Answer from the drawing. Dimensions are ordinates in mm from the lowest x, y and z of the part. A direction names the side the tool comes from. Give positions to 0.01 mm unless a question says otherwise; leave off trailing zeros. Order: outer loops, then holes, each group sorted by start corner. A loop starts at its lowest first (then second) coordinate and runs counter-clockwise, first axis right, second up.
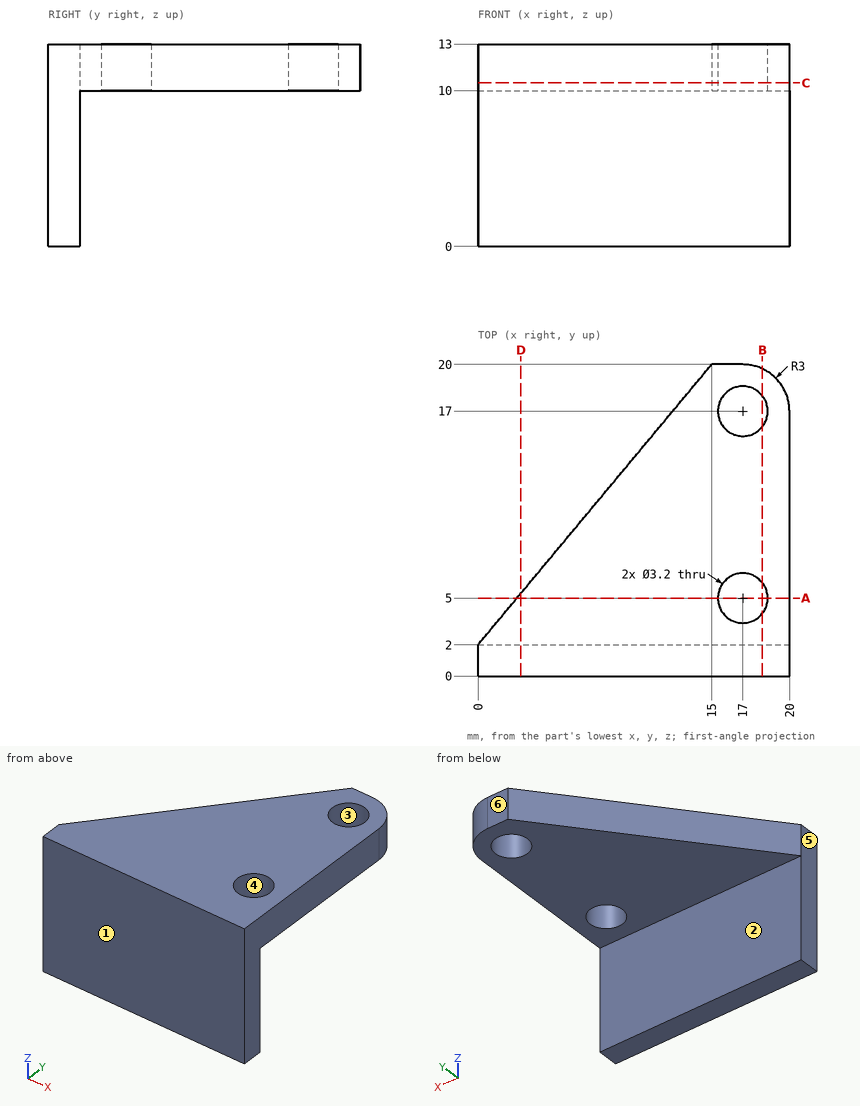
1) Consider L1, parallel to Y at x = 17, z = 12.2; L2, parallel to Y at x = 5.5, z = 4; L3, parallel to Z at x = 13, y = 11.5. Determine where each line is inside the solid, lowest interval first.
Final values:
L1: y = 0 to 3.4, 6.6 to 15.4, 18.6 to 20
L2: y = 0 to 2
L3: z = 10 to 13
2) The part is cut by section A-A on y = 5. Determine the outline of the cut face in (x, z), and give its area (3 significant figures).
Final values:
outline: (2.5, 10) - (15.4, 10) - (15.4, 13) - (2.5, 13) - close; (18.6, 10) - (20, 10) - (20, 13) - (18.6, 13) - close
area: 42.9 mm2
3) A tool of negligible diameter and unlimited length cuts with its end or side. For the marked faces 1 and 2, from which of +Z, -Z, +X, -X, +Y, -Y can it reach the whole face along a straight path? Write none if from no direction.
Final values:
face 1: +Z, -Z, +X, -X, -Y
face 2: -Z, +X, -X, +Y
4) The part is cut by section B-B on x = 18.25. Determine the outline of the cut face in (y, z).
Final values:
outline: (0, 0) - (2, 0) - (2, 10) - (4, 10) - (4, 13) - (0, 13) - close; (6, 10) - (16, 10) - (16, 13) - (6, 13) - close; (18, 10) - (19.73, 10) - (19.73, 13) - (18, 13) - close
5) The part is cut by section D-D on x = 2.75. Determine the outline of the cut face in (y, z).
Final values:
outline: (0, 0) - (2, 0) - (2, 10) - (5.3, 10) - (5.3, 13) - (0, 13) - close
6) The part is cut by section C-C on z = 10.5. Determine the outline of the cut face in (x, y).
Final values:
outline: (0, 0) - (20, 0) - (20, 17) arc R3 ccw to (17, 20) - (15, 20) - (0, 2) - close; hole circle Ø3.2 at (17, 5); hole circle Ø3.2 at (17, 17)
7) For a pull along Y with two mould halves and no side action, classify the marked faces 3, 4, 5 and 6 as released by +Y, released by -Y, zero draft, split by the parting line, or undercut.
Final values:
face 3: undercut
face 4: undercut
face 5: zero draft
face 6: released by +Y
8) Given pin 1 (3.5 mm diameter, centred on x = 17, y = 17, fed in from -Z); pin 2 (2 mm diameter, centred on y = 14, z = 11, fed in from -X), each flat-ended and moving along its own axis, determine where each tip first touches the part or whether it passes through.
Final values:
pin 1: stops at z = 10
pin 2: stops at x = 9.17
